Work out the finished part from the listing and answer in its coordinate system (mm). A direction names the side the tool comes from. Give positions to 0.01 mm unless a question says otherwise; leave off trailing zeros. Order: outer loops, then holes, each group sorted by start corner. A loop starts at its lowest first (then second) coordinate and runs counter-clockwise, first axis right, second up.
```python
from build123d import *

# Parameters (mm, degrees)
CUT_EXTRUDE1_DEPTH = 3
FILLET3_R          = 0.8
CHAMFER1_SIZE      = 0.5
FILLET4_R          = 0.25


with BuildPart() as part:
    # Sketch1 → Revolve1 (revolve)
    with BuildSketch(Plane.XY, mode=Mode.PRIVATE) as revolve1_sk:
        Polygon((0, 0), (5, 0), (5, -6), (3, -6), (3, -16), (0, -16), align=None)
    revolve(revolve1_sk.sketch.rotate(Axis((0, -21, 0), (0, 1, 0)), 90), axis=Axis((0, -21, 0), (0, 1, 0)))

    # Sketch2 → Cut-Extrude1 (cut)
    with BuildSketch(Plane(origin=(0, 0, 0), x_dir=(1, 0, 0), z_dir=(0, 1, 0))):
        Polygon((2.886751346, 0), (1.443375673, 2.5), (-1.443375673, 2.5), (-2.886751346, 0), (-1.443375673, -2.5), (1.443375673, -2.5), align=None)
    extrude(amount=-CUT_EXTRUDE1_DEPTH, mode=Mode.SUBTRACT)

    # Fillet3
    fillet3_edges = [part.edges().sort_by_distance(p)[0] for p in [
        (0, 0, 5),
    ]]
    fillet(fillet3_edges, radius=FILLET3_R)

    # Chamfer1
    chamfer1_edges = [part.edges().sort_by_distance(p)[0] for p in [
        (0, -16, 3),
    ]]
    chamfer(chamfer1_edges, length=CHAMFER1_SIZE)

    # Fillet4
    fillet4_edges = [part.edges().sort_by_distance(p)[0] for p in [
        (0, -6, 3),
        (0, -6, 5),
    ]]
    fillet(fillet4_edges, radius=FILLET4_R)


solid = part.part
```
1. The mould has two halves that part along Z. Classify faces 3 (the face through (0, -1, 2.5)), 4 (the face through (2.155, -1.479, 1.267)), 5 (the face through (3, -6, -2)), 6 (the face through (-0.9, -10.94, -2.86)): pulls with the +Z half, pulls with the -Z half, needs draft (parallel to the pull), parting line crosses it, or undercut.
Findings below:
face 3: undercut
face 4: undercut
face 5: needs draft
face 6: parting line crosses it
2. The part is cut by section C-C (y = -10). Write down the section's boundary in (x, z), then the cut area to 3 significant figures.
Findings below:
outline: circle Ø6 at (0, 0)
area: 28.3 mm2
3. Which of the six approach directions +Z, -Z, +X, -X, +Y, -Y give full straight-line access (tool end or side, diameter ignored) to faces 1 (the face through (-2, 0, 2)), 2 (the face through (-2.175, -1.479, 1.233))?
Findings below:
face 1: +Z, -Z, +X, -X, +Y
face 2: +Y
4. Straight lines are drawn through the part: probe 1 along Y at (x, z) = (-2.5, 2.75); probe 2 along X at (y, z) = (-4.5, -4); probe 3 along Y at (x, z) = (2, 0.25). For each, find the intervals that lie inside material, in ascending order.
Findings below:
probe 1: y = -6 to 0
probe 2: x = -3 to 3
probe 3: y = -16 to -3
5. The part is cut by section B-B (x = 0). Write down the section's boundary in (y, z), then the cut area to 3 significant figures.
Findings below:
outline: (-16, -2.5) - (-15.5, -3) - (-6.25, -3) arc R0.25 cw to (-6, -3.25) - (-6, -4.75) arc R0.25 ccw to (-5.75, -5) - (-0.8, -5) arc R0.8 ccw to (0, -4.2) - (0, -2.5) - (-3, -2.5) - (-3, 2.5) - (0, 2.5) - (0, 4.2) arc R0.8 ccw to (-0.8, 5) - (-5.75, 5) arc R0.25 ccw to (-6, 4.75) - (-6, 3.25) arc R0.25 cw to (-6.25, 3) - (-15.5, 3) - (-16, 2.5) - close
area: 104 mm2
6. Given P1, Ø6, axis at y = -8, z = 2.5, coming from the -X side; P2, Ø1.5, axis at y = -10, z = 3.5, coming from the -X side; P3, Ø1.5, axis at y = -8.5, z = -1, coming from the +X side, each flat-ended and moving along its own axis, determine where each tip first touches the part or whether it passes through.
Findings below:
P1: stops at x = -4.97
P2: stops at x = -1.2
P3: stops at x = 2.99
7. The part is cut by section A-A (y = -2). Write down the section's boundary in (x, z), then the cut area to 3 significant figures.
Findings below:
outline: circle Ø10 at (0, 0); hole (-2.89, 0) - (-1.44, -2.5) - (1.44, -2.5) - (2.89, 0) - (1.44, 2.5) - (-1.44, 2.5) - close
area: 56.9 mm2
8. The part is cut by section D-D (y = -5.5). Write down the section's boundary in (x, z).
Findings below:
outline: circle Ø10 at (0, 0)
